Source: CAD feature listing. Evaluate the final solid. Frame: model axes, mm. A direction names the side the tool comes from. Round coordinates to 2 decimals unless told otherwise and drop trailing zeros. Loops run counter-clockwise (first coordinate to the right, second up) from the corner with the lowest first, then second, coordinate; pieces in that order, holes last. Notation, with made-up numbers: M 50.25,36 L 55.25,36 A14 cw 55.25,56 Z; hole C -11.75,69.25 d3. An arc over 180 degrees is marked long. One line per item, written item: value.
from build123d import *

# Parameters (mm, degrees)
CYLINDER_R             = 12.7
CYLINDER_DEPTH         = 101.6
CYLINDER_ROLL_ANGLE    = 90
SKETCH006_R            = 14.2875
PAD006_DEPTH           = 273.05
SKETCH007_W            = 57.15
SKETCH007_H            = 57.15
PAD007_DEPTH           = 28.575
SKETCH008_R            = 12.7
PAD008_DEPTH           = 9.525
LINEARPATTERN001_COUNT = 2
LINEARPATTERN001_PITCH = 47.625
SKETCH010_R            = 7.9375
PAD010_DEPTH           = 257.175
ARRAY_X_COUNT          = 2
ARRAY_X_PITCH          = 54.61
ARRAY_Y_COUNT          = 2
ARRAY_Y_PITCH          = 54.61
SKETCH_W               = 76.2
SKETCH_H               = 76.2
SKETCH_R               = 7.9375
PAD_DEPTH              = 12.7
PAD001_DEPTH           = 14.2875
SKETCH002_R            = 12.7
PAD002_DEPTH           = 15.875
LINEARPATTERN_COUNT    = 2
LINEARPATTERN_PITCH    = 44.45
SKETCH003_R            = 28.575
SKETCH003_R_2          = 25.4
PAD003_DEPTH           = 203.2
SKETCH004_W            = 76.2
SKETCH004_H            = 76.2
SKETCH004_R            = 7.9375
SKETCH004_R_2          = 25.4
PAD004_DEPTH           = 12.7
SKETCH005_R            = 14.2875
PAD005_DEPTH           = 17.145


with BuildPart() as cylinder:
    # Cylinder → Cylinder (new body)
    with BuildSketch(Plane.XY):
        Circle(CYLINDER_R)
    extrude(amount=CYLINDER_DEPTH)


with BuildPart() as cylinder_1:
    # Cylinder roll: moved
    add(cylinder.part.rotate(Axis((0, 0, 0), (1, 0, 0)), CYLINDER_ROLL_ANGLE))


with BuildPart() as cylinder_2:
    # Cylinder placement: moved
    add(cylinder_1.part.moved(Location((0, -83.82, 83.82))))


with BuildPart() as cylinder001:
    # Clone base: copy of Cylinder
    add(cylinder_2.part)


with BuildPart() as cylinder001_1:
    # Clone placement: moved
    add(cylinder001.part.moved(Location((0, 1.5875, -565.15))))


with BuildPart() as body001:
    # Sketch006 → Pad006 (new body)
    with BuildSketch(Plane.XY):
        Circle(SKETCH006_R)
    extrude(amount=-PAD006_DEPTH)

    # Sketch007 (on Face3 of Pad006) → Pad007 (join)
    with BuildSketch(Plane(origin=(0, 0, -273.05), x_dir=(1, 0, 0), z_dir=(0, 0, -1))):
        Rectangle(SKETCH007_W, SKETCH007_H)
    extrude(amount=-PAD007_DEPTH)

    # Sketch008 (on Face4 of Pad007) → Pad008 (join)
    with BuildSketch(Plane.XZ.offset(28.575)):
        with BuildLine():
            Line((-25.4, -247.65), (25.4, -247.65))
            Line((25.4, -247.65), (25.4, -328.929945))
            ThreePointArc((-25.4, -328.929945), (0, -354.33), (25.4, -328.929945))
            Line((-25.4, -328.929945), (-25.4, -247.65))
        make_face()
        with Locations((0, -328.93)):
            Circle(SKETCH008_R, mode=Mode.SUBTRACT)
    pad008 = extrude(amount=-PAD008_DEPTH)

    # LinearPattern001: Pad008 ×2
    with Locations(*[(0, i * LINEARPATTERN001_PITCH, 0) for i in range(1, LINEARPATTERN001_COUNT)]):
        add(pad008)


with BuildPart() as body001_1:
    # Body001 placement: moved
    add(body001.part.moved(Location((0, 0, -152.4))))


with BuildPart() as array:
    # Sketch010 → Pad010 (new body)
    with BuildSketch(Plane.XY):
        with Locations((26.9875, -26.9875)):
            Circle(SKETCH010_R)
    extrude(amount=-PAD010_DEPTH)

    # Array X: Array ×2


with BuildPart() as array_1:
    add(array.part)
    with Locations(*[(-i * ARRAY_X_PITCH, 0, 0) for i in range(1, ARRAY_X_COUNT)]):
        add(array.part)

    # Array Y: Array ×2


with BuildPart() as array_2:
    add(array_1.part)
    with Locations(*[(0, i * ARRAY_Y_PITCH, 0) for i in range(1, ARRAY_Y_COUNT)]):
        add(array_1.part)


with BuildPart() as array_3:
    # Array placement: moved
    add(array_2.part.moved(Location((0, 0, 25.4))))


with BuildPart() as fusion:
    # Sketch → Pad (new body)
    with BuildSketch(Plane.XY):
        Rectangle(SKETCH_W, SKETCH_H)
        with Locations((-26.9875, 26.9875)):
            Circle(SKETCH_R, mode=Mode.SUBTRACT)
        with Locations((26.9875, 26.9875)):
            Circle(SKETCH_R, mode=Mode.SUBTRACT)
        with Locations((-26.9875, -26.9875)):
            Circle(SKETCH_R, mode=Mode.SUBTRACT)
        with Locations((26.9875, -26.9875)):
            Circle(SKETCH_R, mode=Mode.SUBTRACT)
    extrude(amount=PAD_DEPTH)

    # Sketch001 → Pad001 (join, symmetric)
    with BuildSketch(Plane(origin=(0, 0, 12.7), x_dir=(1, 0, 0), z_dir=(0, -1, 0))):
        Polygon((-38.1, 0), (38.1, 0), (22.225, 19.05), (-22.225, 19.05), align=None)
    extrude(amount=PAD001_DEPTH, both=True)

    # Sketch002 (on Face15 of Pad001) → Pad002 (join)
    with BuildSketch(Plane.XZ.offset(14.2875)):
        with BuildLine():
            Line((-17.4625, 0), (17.4625, 0))
            Line((17.4625, 0), (17.4625, 65.374917))
            ThreePointArc((17.4625, 65.374917), (0, 109.22), (-17.4625, 65.374917))
            Line((-17.4625, 65.374917), (-17.4625, 0))
        make_face()
        with Locations((0, 83.82)):
            Circle(SKETCH002_R, mode=Mode.SUBTRACT)
    pad002 = extrude(amount=PAD002_DEPTH)

    # LinearPattern: Pad002 ×2
    with Locations(*[(0, i * LINEARPATTERN_PITCH, 0) for i in range(1, LINEARPATTERN_COUNT)]):
        add(pad002)

    # Sketch003 (on Face4 of LinearPattern) → Pad003 (join)
    with BuildSketch(Plane(origin=(0, 0, 0), x_dir=(1, 0, 0), z_dir=(0, 0, -1))):
        Circle(SKETCH003_R)
        Circle(SKETCH003_R_2, mode=Mode.SUBTRACT)
    extrude(amount=PAD003_DEPTH)

    # Sketch004 (on Face28 of Pad003) → Pad004 (join)
    with BuildSketch(Plane(origin=(0, 0, -203.2), x_dir=(1, 0, 0), z_dir=(0, 0, -1))):
        Rectangle(SKETCH004_W, SKETCH004_H)
        with Locations((-26.9875, 26.9875)):
            Circle(SKETCH004_R, mode=Mode.SUBTRACT)
        with Locations((26.9875, 26.9875)):
            Circle(SKETCH004_R, mode=Mode.SUBTRACT)
        with Locations((-26.9875, -26.9875)):
            Circle(SKETCH004_R, mode=Mode.SUBTRACT)
        with Locations((26.9875, -26.9875)):
            Circle(SKETCH004_R, mode=Mode.SUBTRACT)
        Circle(SKETCH004_R_2, mode=Mode.SUBTRACT)
    extrude(amount=PAD004_DEPTH)

    # Sketch005 (on Face43 of Pad004) → Pad005 (join)
    with BuildSketch(Plane(origin=(0, 0, -215.9), x_dir=(1, 0, 0), z_dir=(0, 0, -1))):
        with BuildLine():
            ThreePointArc((21.997045, 12.7), (17.960512, 17.960512), (12.7, 21.997045))
            Line((12.7, 34.697045), (12.7, 21.997045))
            Line((-12.7, 34.697045), (12.7, 34.697045))
            Line((-12.7, 21.997045), (-12.7, 34.697045))
            ThreePointArc((-12.7, 21.997045), (-17.960512, 17.960512), (-21.997045, 12.7))
            Line((-34.697045, 12.7), (-21.997045, 12.7))
            Line((-34.697045, -12.7), (-34.697045, 12.7))
            Line((-21.997045, -12.7), (-34.697045, -12.7))
            ThreePointArc((-21.997045, -12.7), (-17.960512, -17.960512), (-12.7, -21.997045))
            Line((-12.7, -21.997045), (-12.7, -47.397045))
            Line((-12.7, -47.397045), (12.7, -47.397045))
            Line((12.7, -47.397045), (12.7, -21.997045))
            ThreePointArc((12.7, -21.997045), (17.960512, -17.960512), (21.997045, -12.7))
            Line((21.997045, -12.7), (34.697045, -12.7))
            Line((34.697045, -12.7), (34.697045, 12.7))
            Line((34.697045, 12.7), (21.997045, 12.7))
        make_face()
        Circle(SKETCH005_R, mode=Mode.SUBTRACT)
    extrude(amount=PAD005_DEPTH)

    # Fusion: union Body001, Array
    add(body001_1.part)
    add(array_3.part)


with BuildPart() as fusion_1:
    # Fusion placement: moved
    add(fusion.part.moved(Location((0, -133.0325, 0))))


with BuildPart() as body003:
    # Fusion001 base: copy of Cylinder
    add(cylinder_2.part)

    # Fusion001: union Cylinder001, Fusion
    add(cylinder001_1.part)
    add(fusion_1.part)


with BuildPart() as body003_1:
    # Body003 placement: moved
    add(body003.part.moved(Location((0, -100, 0))))


solid = body003_1.part
1. Ray query, line 1 (Z direction, x = -22, y = -242.5) (3 decimals); line 2 (Z direction, x = 0, y = -211) (3 decimals); line 3 (Y direction, x = 0, z = -163) (1 decimal). Return the intervals inside material, ascending. Write a range as [from, to].
Report:
line 1: z = [-425.45, -396.875], [-233.045, -215.9], [0, 31.75]
line 2: z = [-506.73, -396.875], [-233.045, -215.9], [0, 109.22]
line 3: y = [-261.6, -258.4], [-247.3, -218.7], [-207.6, -204.5]
2. Pin query (flat end, axial travel): pin 1 (23 mm diameter, centred on x = -15.5, y = -248, fed in from +Z); pin 2 (3 mm diameter, centred on y = -257.5, z = -456.5, fed in from +X); pin 3 (3 mm diameter, centred on x = 0.5, y = -189.5, fed in from +Z). Return the tip coordinate at first contact, or that it passes through.
Report:
pin 1: stops at z = 108.9
pin 2: stops at x = 25.4
pin 3: stops at z = 96.52
3. Section query D-D (z = 83.82). Return the cut outline in (x, y) (3 decimals), and give its area (3 significant figures).
Report:
outline: M -25.4,-263.195 L -12.7,-263.195 L -12.7,-285.42 L 12.7,-285.42 L 12.7,-263.195 L 25.4,-263.195 L 25.4,-247.32 L 12.7,-247.32 L 12.7,-218.745 L 25.4,-218.745 L 25.4,-202.87 L 12.7,-202.87 L 12.7,-183.82 L -12.7,-183.82 L -12.7,-202.87 L -25.4,-202.87 L -25.4,-218.745 L -12.7,-218.745 L -12.7,-247.32 L -25.4,-247.32 Z
area: 3,390 mm2
4. Reachability of faces 1 (the face through (-26, -247.32, 20)), 2 (the face through (-6.194, -205.137, -100.178)), 3 (the face through (-34.697, -233, -224)), 4 (the face through (-28, -205, 25.4)), 5 (the face through (0, -233, 31.75)) from +Z, -Z, +X, -X, +Y, -Y: full face, straight path, thin tool, end or side. Return the list, or none.
Report:
face 1: -X
face 2: none
face 3: -Z, -X
face 4: -X, +Y
face 5: +X, -X
5. Section query A-A (z = -223). Return the cut outline in (x, y) (1 decimal).
Report:
outline: C -27.6,-260 d15.9; C -27.6,-205.4 d15.9; M -34.7,-245.7 L -22,-245.7 A25.4 ccw -12.7,-255 L -12.7,-267.7 L 12.7,-267.7 L 12.7,-255 A25.4 ccw 22,-245.7 L 34.7,-245.7 L 34.7,-220.3 L 22,-220.3 A25.4 ccw 12.7,-211 L 12.7,-185.6 L -12.7,-185.6 L -12.7,-211 A25.4 ccw -22,-220.3 L -34.7,-220.3 Z; C 27,-260 d15.9; C 27,-205.4 d15.9
6. Pull-direction query (X, two-part tool) for faces 6 (the face through (0, -233, 0)), 7 (the face through (-25.4, -257, -454)), 8 (the face through (-1.653, -272.564, -468.738)); classes: released by +X, released by -X, zero draft, split by the parting line, or undercut.
Report:
face 6: undercut
face 7: released by -X
face 8: split by the parting line
7. Section query B-B (z = -57). Count the separate pieces of the cut face and the enclosed holes in it, and give its area (3 significant figures).
Report:
separate pieces: 5
enclosed holes: 1
area: 1,330 mm2
